Check sheet for the drawn part. Datum: minimum x, y, z corner. Units: mm. A direction names the side the tool comes from. Round coordinates to 2 decimals unless told otherwise and drop trailing zeros. Write each loop counter-clockwise with the first axis right and the second up, starting at its lowest first coordinate (ties: lowest second). Pieces come first, ordered by that corner, then holes. Notation, with made-up numbers: (89, 40) - (135, 40) arc R18 cw to (135, 51) - close; hole circle Ø9 at (19, 1.5). An arc over 180 degrees is marked (long way). Answer as a JSON object with one key per item and string values.
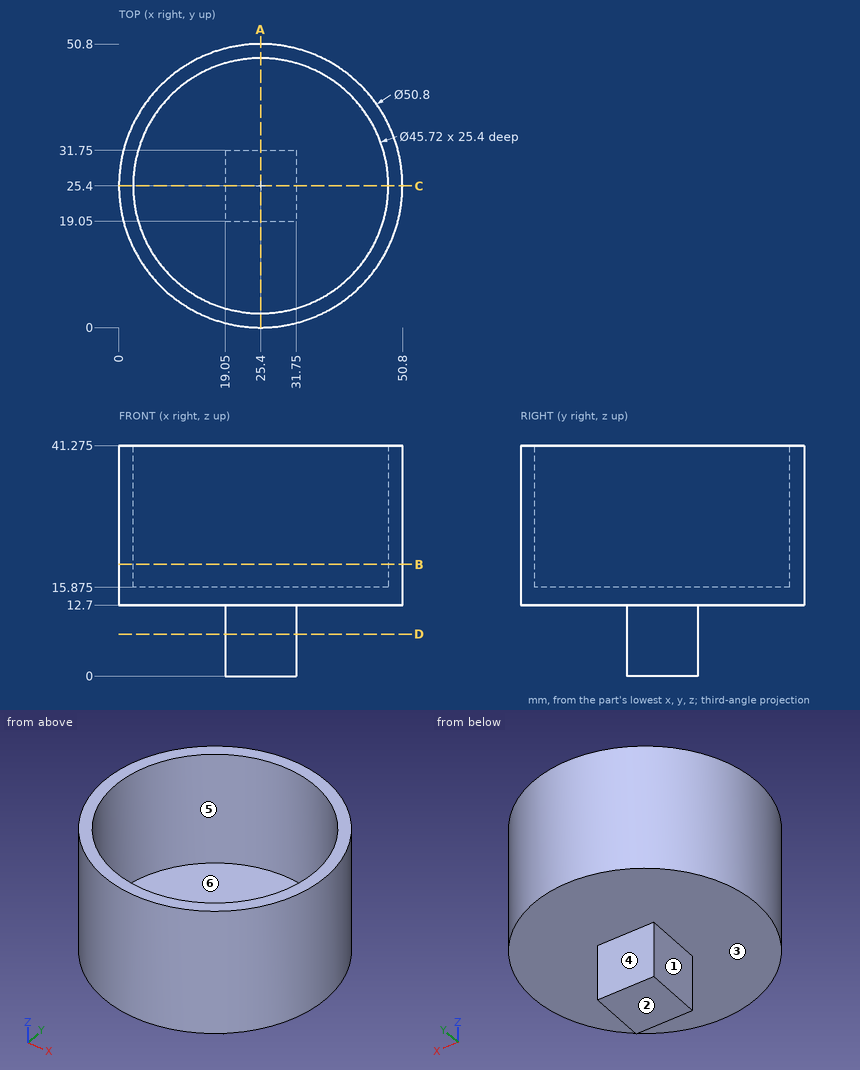
1. Cross-section at D-D (z = 7.5). Record the boundary of the cut face in (x, y).
Completed:
{"outline": "(19.05, 19.05) - (31.75, 19.05) - (31.75, 31.75) - (19.05, 31.75) - close"}
2. Access from +Z, -Z, +X, -X, +Y, -Y to the whole of each face (thin tool, end or side, straight path). Record for the marked faces 1 and 2.
Completed:
{"face 1": "-Z, -X, +Y, -Y", "face 2": "-Z, +X, -X, +Y, -Y"}
3. Mould release check, pull along Y, two halves, no side actions. Record for the marked faces 3, 4, 5 and 6: released by +Y, released by -Y, zero draft, split by the parting line, or undercut.
Completed:
{"face 3": "zero draft", "face 4": "released by +Y", "face 5": "undercut", "face 6": "undercut"}
4. Material ranges on probe 1 along Y at (x, z) = (25, 24); probe 2 along Z at (x, y) = (31, 21.5) (3 decimals), recorded low to high. Write a range as from..to.
Completed:
{"probe 1": "y = 0..2.54, 48.26..50.8", "probe 2": "z = 0..15.875"}
5. Go/stop test with flat-tipped pins: pin 1 (8 mm diameter, centred on y = 38.5, z = 18, fed in from +X); pin 2 (2 mm diameter, centred on x = 18.5, z = 33, fed in from +Y); pin 3 (6.5 mm diameter, centred on y = 28, z = 9, fed in from -X); pin 4 (5 mm diameter, centred on x = 45.5, z = 8.5, fed in from +Y). Record where each tip stops, or that it passes through.
Completed:
{"pin 1": "stops at x = 49.11", "pin 2": "stops at y = 50.11", "pin 3": "stops at x = 19.05", "pin 4": "passes through"}
6. Cross-section at B-B (z = 20). Record the boundary of the cut face in (x, y), plus the area to 3 significant figures.
Completed:
{"outline": "circle Ø50.8 at (25.4, 25.4); hole circle Ø45.72 at (25.4, 25.4)", "area": "385 mm^2"}
7. Cross-section at A-A (x = 25.4). Record the boundary of the cut face in (y, z) (3 decimals).
Completed:
{"outline": "(0, 12.7) - (19.05, 12.7) - (19.05, 0) - (31.75, 0) - (31.75, 12.7) - (50.8, 12.7) - (50.8, 41.275) - (48.26, 41.275) - (48.26, 15.875) - (2.54, 15.875) - (2.54, 41.275) - (0, 41.275) - close"}
